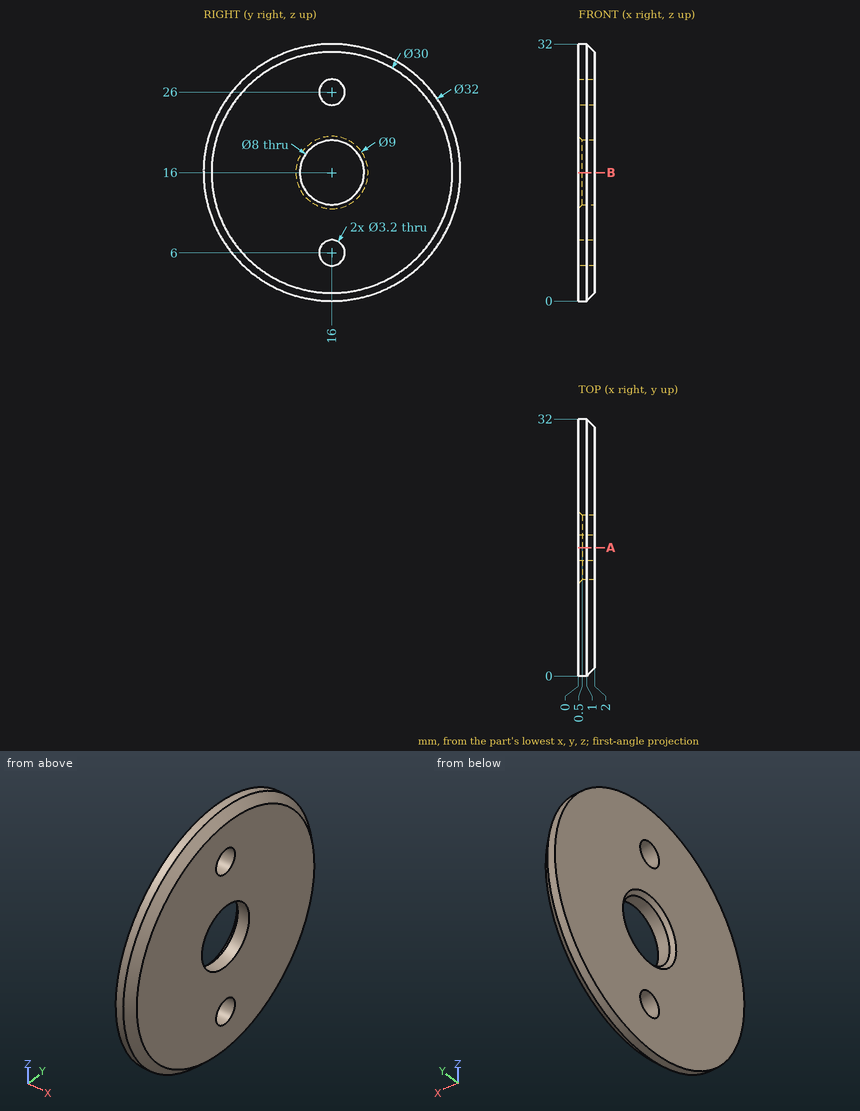
Could you check a few things on this drawing? It's one solid part, dimensions in mm from its lowest x, y, z. Give positions to 0.01 mm unless a question says otherwise; leave off trailing zeros. Order: outer loops, then holes, each group sorted by start corner. A loop starts at its lowest first (then second) coordinate and runs counter-clockwise, first axis right, second up. Notation, with made-up numbers: (51, 10) - (94, 10) arc R34 ccw to (94, 45) - close; hole circle Ø1 at (83, 72.25). An arc over 180 degrees is marked (long way). Answer as a JSON object with one key per item and string values. Group by question number.
Item 1: If we section it at B-B on z = 16: Please give me the cut outline in (x, y).
Item 2: For P1, Ø1, axis at x = 2, z = 8, coming from the -Y side; P2, Ø13, axis at y = 16, z = 16, coming from the +X side, each with a flat end and sliding along its axis, tell me the tip position at first contact or that it passes through.
Item 3: Please list where these lines run through material, in increasing order: probe 1 along Z at (x, y) = (0.6, 16.5); probe 2 along Y at (x, z) = (0.9, 16); probe 3 along Y at (x, z) = (1.05, 16).
Item 4: If we section it at A-A on y = 16: Please give me the cut outline in (x, z).
Result set:
{
 "1": {"outline": "(0, 0) - (1, 0) - (2, 1) - (2, 12) - (0.5, 12) - (0, 11.5) - close; (0, 20.5) - (0.5, 20) - (2, 20) - (2, 31) - (1, 32) - (0, 32) - close"},
 "2": {"P1": "y = 2.65", "P2": "x = 2"},
 "3": {"probe 1": "0.01 to 4.48, 7.52 to 12.03, 19.97 to 24.48, 27.52 to 31.99", "probe 2": "0 to 12, 20 to 32", "probe 3": "0.05 to 12, 20 to 31.95"},
 "4": {"outline": "(0, 0) - (1, 0) - (2, 1) - (2, 4.4) - (0, 4.4) - close; (0, 7.6) - (2, 7.6) - (2, 12) - (0.5, 12) - (0, 11.5) - close; (0, 20.5) - (0.5, 20) - (2, 20) - (2, 24.4) - (0, 24.4) - close; (0, 27.6) - (2, 27.6) - (2, 31) - (1, 32) - (0, 32) - close"}
}
